from build123d import *

# Parameters (mm, degrees)
SKETCH1_W          = 600
SKETCH1_H          = 650
SKETCH1_R          = 152.4
SKETCH1_R_2        = 5
BASE_FLANGE1_DEPTH = 1.2


# Sheet-metal steps are written as plain solids
with BuildPart() as part:
    # Sketch1 → Base-Flange1 (new body)
    with BuildSketch(Plane.XY):
        Rectangle(SKETCH1_W, SKETCH1_H)
        Circle(SKETCH1_R, mode=Mode.SUBTRACT)
        with Locations((43.662772909, 162.951686895)):
            Circle(SKETCH1_R_2, mode=Mode.SUBTRACT)
        with Locations((119.288913986, 119.288913986)):
            Circle(SKETCH1_R_2, mode=Mode.SUBTRACT)
        with Locations((162.951686895, 43.662772909)):
            Circle(SKETCH1_R_2, mode=Mode.SUBTRACT)
        with Locations((162.951686895, -43.662772909)):
            Circle(SKETCH1_R_2, mode=Mode.SUBTRACT)
        with Locations((119.288913986, -119.288913986)):
            Circle(SKETCH1_R_2, mode=Mode.SUBTRACT)
        with Locations((43.662772909, -162.951686895)):
            Circle(SKETCH1_R_2, mode=Mode.SUBTRACT)
        with Locations((-43.662772909, -162.951686895)):
            Circle(SKETCH1_R_2, mode=Mode.SUBTRACT)
        with Locations((-119.288913986, -119.288913986)):
            Circle(SKETCH1_R_2, mode=Mode.SUBTRACT)
        with Locations((-162.951686895, -43.662772909)):
            Circle(SKETCH1_R_2, mode=Mode.SUBTRACT)
        with Locations((-162.951686895, 43.662772909)):
            Circle(SKETCH1_R_2, mode=Mode.SUBTRACT)
        with Locations((-119.288913986, 119.288913986)):
            Circle(SKETCH1_R_2, mode=Mode.SUBTRACT)
        with Locations((-43.662772909, 162.951686895)):
            Circle(SKETCH1_R_2, mode=Mode.SUBTRACT)
    extrude(amount=-BASE_FLANGE1_DEPTH)


solid = part.part
Build history of the part. All positions in model axes, mm. Coordinates: 2 decimals unless noted, no trailing zeros. Order: outer loops, then holes, each group sorted by start corner. A loop starts at its lowest first (then second) coordinate and runs counter-clockwise, first axis right, second up. Notation, with made-up numbers: (36, 39.5) - (40, 39.5) arc R17 ccw to (40, 43.5) - close; hole circle Ø8 at (-25.5, 43.25). An arc over 180 degrees is marked (long way). Write item = value, one per line. Start each with the question number.
1) Saw through at B-B on y = 0. Write the cut outline in (x, z), then the cut area to 3 significant figures.
2) Wall check: line 1 along Y through (x, z) = (120, -0.6); line 2 along X through (y, z) = (116.5, -0.5); line 3 along Y through (x, z) = (164.5, -0.9). Give the ranges that are in metal, low to high. Write a range as from..to.
3) Saw through at A-A on x = 0. Write the cut outline in (y, z).
4) Saw through at C-C on z = -0.9. Count the separate pieces of the cut face and the enclosed holes in it, then the cut area to 3 significant figures.
5) Two-plate mould, pull along X, no slides. Class faces 1 (the face through (-138, 77, -1.2)), 2 (the face through (-120.94, -92.73, -0.59)): pulls with the +X half, pulls with the -X half, needs draft (parallel to the pull), parting line crosses it, or undercut.
From the geometry:
q1.outline = (-300, -1.2) - (-152.4, -1.2) - (-152.4, 0) - (-300, 0) - close; (152.4, -1.2) - (300, -1.2) - (300, 0) - (152.4, 0) - close
q1.area = 354 mm^2
q2.line_1 = -325..-124.24, -114.34..-93.95, 93.95..114.34, 124.24..325
q2.line_2 = -300..-123.44, -115.14..-98.25, 98.25..115.14, 123.44..300
q2.line_3 = -325..-48.42, -38.91..38.91, 48.42..325
q3.outline = (-325, -1.2) - (-152.4, -1.2) - (-152.4, 0) - (-325, 0) - close; (152.4, -1.2) - (325, -1.2) - (325, 0) - (152.4, 0) - close
q4.separate_pieces = 1
q4.enclosed_holes = 13
q4.area = 316,000 mm^2
q5.face_1 = needs draft
q5.face_2 = undercut
